Could you check a few things on this model? Use its own coordinates, in mm. A direction names the side the tool comes from. Coordinates: 2 decimals unless noted, no trailing zeros. Loops run counter-clockwise (first coordinate to the right, second up) from the corner with the lowest first, then second, coordinate; pieces in that order, holes last.
1) Imagine slicing it at C-C on x = 18.5. Please give me the cut outline in (y, z).
2) For faces 4 (the face through (20.91, 38.58, 0.2)), 5 (the face through (14, 152.4, 0)), which set-ups out of +Z, -Z, +X, -X, +Y, -Y let a thin tool reach every point of the face, with its end or its side?
3) Thinking about a two-plate mould opening in X: for faces 1 (the face through (14, 0, 0)), 2 (the face through (-2.517, 75.133, 11.336)), 3 (the face through (20.75, 112.78, 0.2)), which applies, released by +X, released by -X, zero draft, split by the parting line, or undercut?
4) Imagine slicing it at B-B on y = 92.5. Please give me the cut outline in (x, z) (1 decimal), plus the area to 3 significant figures.
5) Imagine slicing it at A-A on z = 0. Please give me the cut outline in (x, y), plus the area to 3 significant figures.
6) Will these pins go through, and if not, where does the flat tip stop? P1, Ø8, axis at y = 32.5, z = 1.5, coming from the +X side; P2, Ø2, axis at y = 20.5, z = 4.5, coming from the -X side; P3, Ø1.5, axis at y = 74, z = -5, coming from the -X side.
7) If I drill on line 1 along Z through (x, y) = (6, 46); line 2 along X through (y, z) = (116, -6.25); line 3 along X through (y, z) = (39, 0), over which ranges is the centre line in solid material (lowest first)?
8) Imagine slicing it at D-D on y = 119. Please give me the cut outline in (x, z) (1 decimal), plus the area to 3 significant figures.
```python
from build123d import *

# Parameters (mm, degrees)
SKETCH1_R           = 14.2875
SKETCH1_R_2         = 11.6125
BOSS_EXTRUDE1_DEPTH = 152.4
SKETCH2_W           = 28.575
SKETCH2_H           = 152.4
BOSS_EXTRUDE2_DEPTH = 12.7
BOSS_EXTRUDE3_DEPTH = 152.4
CUT_EXTRUDE1_DEPTH  = 29.575
FILLET1_R           = 2


with BuildPart() as part:
    # Sketch1 → Boss-Extrude1 (new body)
    with BuildSketch(Plane(origin=(0, 0, 0), x_dir=(1, 0, 0), z_dir=(0, 1, 0))):
        Circle(SKETCH1_R)
        Circle(SKETCH1_R_2, mode=Mode.SUBTRACT)
    extrude(amount=BOSS_EXTRUDE1_DEPTH)



with BuildPart() as body_2:
    # Sketch2 → Boss-Extrude2 (new body)
    with BuildSketch(Plane(origin=(14.2875, 0, 0), x_dir=(0, 0, -1), z_dir=(1, 0, 0))):
        with Locations((0, 76.2)):
            Rectangle(SKETCH2_W, SKETCH2_H)
    extrude(amount=BOSS_EXTRUDE2_DEPTH)


with BuildPart() as part_1:
    add(part.part)

    add(body_2.part)  # Boss-Extrude3 merges body 2
    # Sketch3 → Boss-Extrude3 (add, through all)
    with BuildSketch(Plane(origin=(0, 152.4, 0), x_dir=(1, 0, 0), z_dir=(0, 1, 0))):
        with BuildLine():
            Line((14.2875, -14.2875), (0, -14.2875))
            ThreePointArc((0, -14.2875), (14.2875, 0), (0, 14.2875))
            Line((0, 14.2875), (14.2875, 14.2875))
            Line((14.2875, 14.2875), (26.9875, 14.2875))
            Line((26.9875, 14.2875), (26.9875, -14.2875))
            Line((26.9875, -14.2875), (14.2875, -14.2875))
        make_face()
    extrude(amount=-BOSS_EXTRUDE3_DEPTH)

    # Sketch5 → Cut-Extrude1 (cut, through all)
    with BuildSketch(Plane.XY.offset(14.2875)):
        Polygon((26.9875, 0), (14.9875, 76.2), (26.9875, 152.4), align=None)
    extrude(amount=-CUT_EXTRUDE1_DEPTH, mode=Mode.SUBTRACT)

    # Fillet1
    fillet1_edges = [part_1.edges().sort_by_distance(p)[0] for p in [
        (26.9875, 0, 0),
        (26.9875, 152.4, 0),
        (14.9875, 76.2, 0),
    ]]
    fillet(fillet1_edges, radius=FILLET1_R)


solid = part_1.part
```
Filled in:
1. outline: (0, -14.29) - (53.9, -14.29) - (53.9, 14.29) - (0, 14.29) - close; (98.5, -14.29) - (152.4, -14.29) - (152.4, 14.29) - (98.5, 14.29) - close
2. face 4: +Z, -Z, +X
2. face 5: +Z, -Z, +X, -X, +Y
3. face 1: zero draft
3. face 2: undercut
3. face 3: released by +X
4. outline: (0, -14.3) - (17.6, -14.3) - (17.6, 14.3) - (0, 14.3) arc R14.3 ccw to start; hole circle Ø23.2 at (0, 0)
4. area: 399 mm2
5. outline: (-14.29, 0) - (-11.61, 0) - (-11.61, 152.4) - (-14.29, 152.4) - close; (11.61, 0) - (24.65, 0) arc R2 ccw to (26.62, 2.31) - (15.04, 75.89) arc R2 cw to (15.04, 76.51) - (26.62, 150.09) arc R2 ccw to (24.65, 152.4) - (11.61, 152.4) - close
5. area: 1,830 mm2
6. P1: stops at x = 22.5
6. P2: stops at x = -13.85
6. P3: stops at x = -13.64
7. line 1: z = -14.29 to -9.94, 9.94 to 14.29
7. line 2: x = -12.85 to -9.79, 9.79 to 21.26
7. line 3: x = -14.29 to -11.61, 11.61 to 20.85
8. outline: (0, -14.3) - (21.7, -14.3) - (21.7, 14.3) - (0, 14.3) arc R14.3 ccw to start; hole circle Ø23.2 at (0, 0)
8. area: 518 mm2
